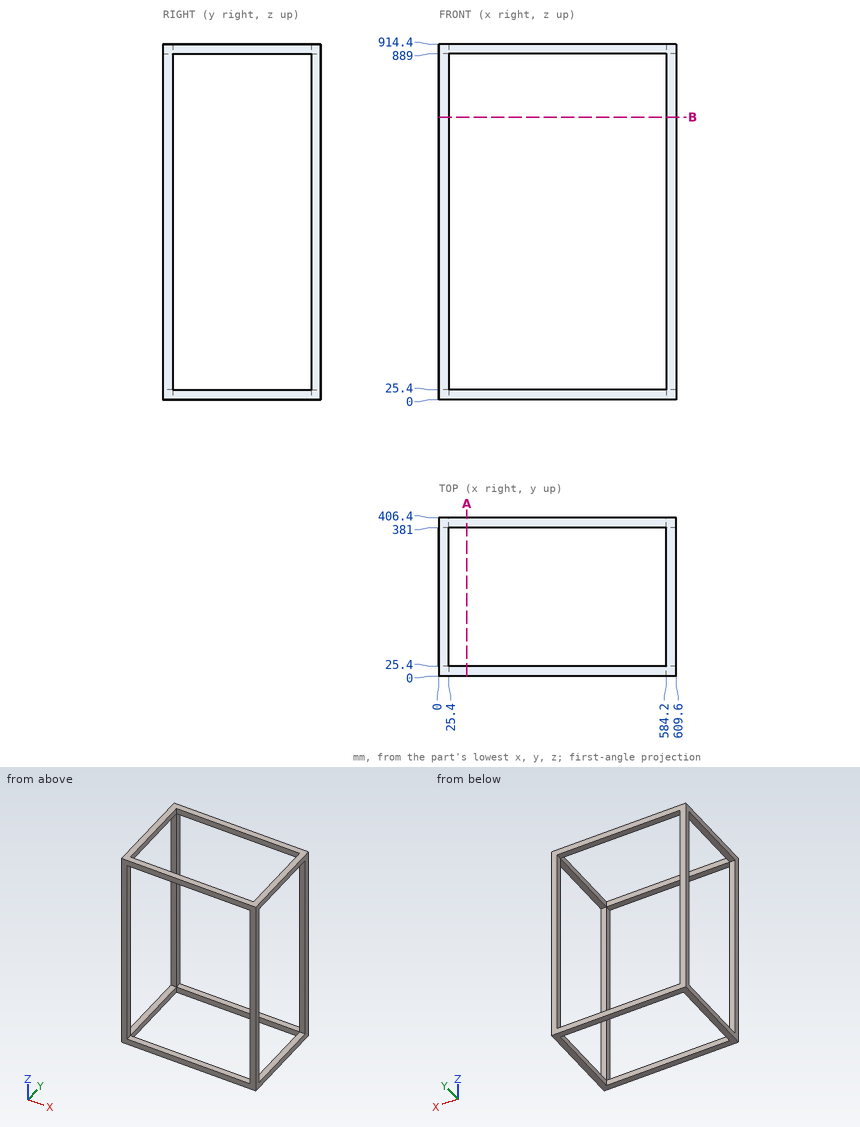
Study the drawing (mm; zero at the part's minimum x, y, z) and answer. Give positions to 0.01 mm unless a question says otherwise; leave off trailing zeros. Write each loop counter-clockwise with the first axis right and the second up, starting at its lowest first coordinate (ties: lowest second). Pieces come first, ordered by that corner, then holes.
Item 1: A flat-ended cylindrical pin translates along its axis: P1, Ø12.5, axis at y = 399.5, z = 382, coming from the -X side. Find the tip coordinate at first contact, or state that the pin passes through.
Item 2: Find the intervals of material crossed by line 1 along Z through (x, y) = (285, 382.5), in increasing order.
Item 3: Section A-A, the plane x = 72 is taken. Write down the section's boundary in (y, z).
Item 4: Section B-B, the plane z = 726.5 is taken. Write down the section's boundary in (x, y), plus the area to 3 significant figures.
Completed:
1. P1: stops at x = 0
2. line 1: z = 0 to 25.4, 889 to 914.4
3. outline: (0, 0) - (25.4, 0) - (25.4, 25.4) - (0, 25.4) - close; (0, 889) - (25.4, 889) - (25.4, 914.4) - (0, 914.4) - close; (381, 0) - (406.4, 0) - (406.4, 25.4) - (381, 25.4) - close; (381, 889) - (406.4, 889) - (406.4, 914.4) - (381, 914.4) - close
4. outline: (0, 0) - (25.4, 0) - (25.4, 25.4) - (0, 25.4) - close; (0, 381) - (25.4, 381) - (25.4, 406.4) - (0, 406.4) - close; (584.2, 0) - (609.6, 0) - (609.6, 25.4) - (584.2, 25.4) - close; (584.2, 381) - (609.6, 381) - (609.6, 406.4) - (584.2, 406.4) - close
4. area: 2,580 mm2
